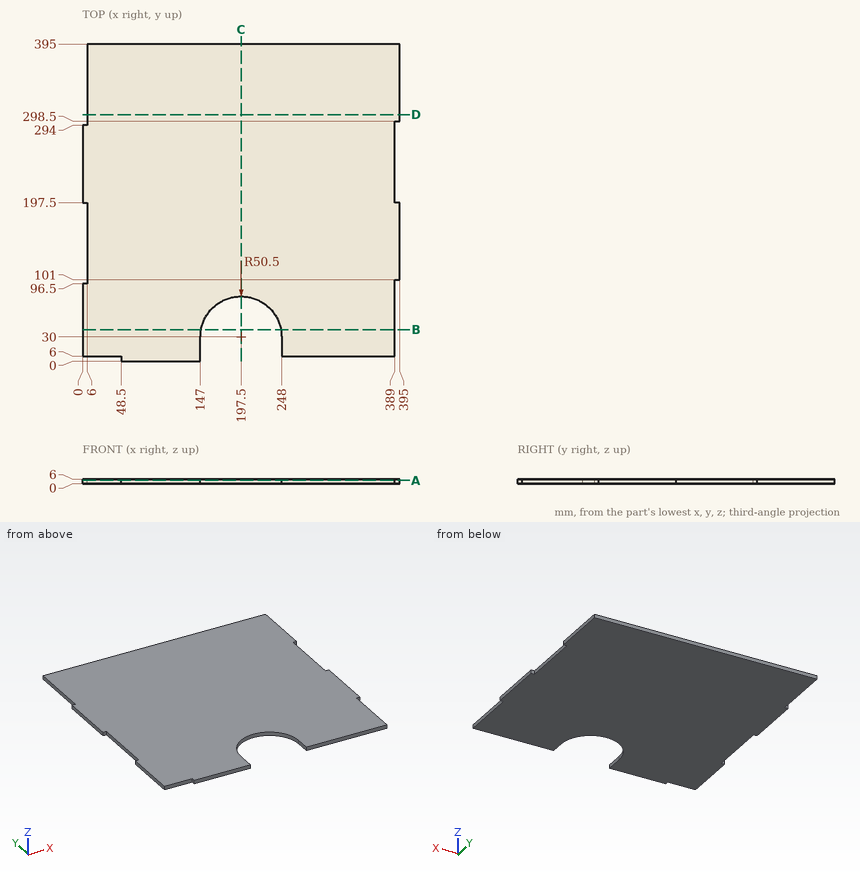
Study the drawing (mm; zero at the part's minimum x, y, z) and answer. Coordinates: 2 decimals unless noted, no trailing zeros. Loops run counter-clockwise (first coordinate to the right, second up) from the corner with the lowest first, then second, coordinate; pieces in that order, holes last. Notation, with made-up numbers: M 42,-3.5 L 60,-3.5 A19 ccw 60,4.5 Z; hole C -25.5,26.25 d3. An arc over 180 degrees is marked long. Answer in a Markdown table with one row per item.
1) Find section D-D (y = 307). Determine the outline of the cut face in (x, z).
Answers below:
| item | result |
|---|---|
| outline | M 6,0 L 395,0 L 395,6 L 6,6 Z |
2) Find section C-C (x = 197.5). Determine the outline of the cut face in (y, z).
Answers below:
| item | result |
|---|---|
| outline | M 80.5,0 L 395,0 L 395,6 L 80.5,6 Z |
3) Given pin 1 (2 mm diameter, centred on y = 58.5, z = 1, fed in from +X); pin 2 (3 mm diameter, centred on x = 286, z = 2.5, fed in from -Y); pin 3 (1.8 mm diameter, centred on y = 1.5, z = 4.5, fed in from -X), each flat-ended and moving along its own axis, determine where each tip first touches the part or whether it passes through.
Answers below:
| item | result |
|---|---|
| pin 1 | x = 389 |
| pin 2 | y = 6 |
| pin 3 | x = 48.5 |
4) Find section A-A (z = 4.25). Determine the outline of the cut face in (x, y).
Answers below:
| item | result |
|---|---|
| outline | M 0,6 L 48.5,6 L 48.5,0 L 147,0 L 147,30 A50.5 cw 248,30 L 248,6 L 389,6 L 389,101 L 395,101 L 395,197.5 L 389,197.5 L 389,298.5 L 395,298.5 L 395,395 L 6,395 L 6,294 L 0,294 L 0,197.5 L 6,197.5 L 6,96.5 L 0,96.5 Z |
5) Find section B-B (y = 39). Determine the outline of the cut face in (x, z), then the cut area to 3 significant figures.
Answers below:
| item | result |
|---|---|
| outline | M 0,0 L 147.81,0 L 147.81,6 L 0,6 Z; M 247.19,0 L 389,0 L 389,6 L 247.19,6 Z |
| area | 1,740 mm^2 |
6) Find the intervals of material crossed by probe 1 along X at (y, z) = (107, 3); probe 2 along X at (y, z) = (28, 2.8), in increasing order.
Answers below:
| item | result |
|---|---|
| probe 1 | 6 to 395 |
| probe 2 | 0 to 147, 248 to 389 |
